Work out the finished part from the listing and answer in its coordinate system (mm). Round coordinates to 2 decimals unless told otherwise and drop trailing zeros.
from build123d import *

# Parameters (mm, degrees)
F1_DEPTH = 200
F4_T     = -0.6
F3_W     = 0.2
F3_H     = 14
F5_DEPTH = 25
F6_W     = 0.2
F6_H     = 14
F7_DEPTH = 25
F8_R     = 0.4


with BuildPart() as f1:
    # F0 (on Right) → F1 (new body)
    with BuildSketch(Plane.YZ):
        with BuildLine():
            add(Edge.make_bspline(
                [(18.4494327754, -3.8520128001), (15.5609515421, -0.4847487874), (8.1340167717, 2.2164674432), (-12.2966120419, 0.5504568669), (-24.9624218007, -2.9072897866), (-31.5505672246, -3.8520128001)],
                knots=[0, 0, 0, 0, 0.2747109337, 0.6355042516, 1, 1, 1, 1], degree=3))
            Line((-31.5505672246, -3.8520128001), (18.4494327754, -3.8520128001))
        make_face()
    extrude(amount=F1_DEPTH)


with BuildPart() as f1_1:
    # F2: moved
    add(f1.part.moved(Location((-100, 0, 16.3))))

    # F4
    f4_openings = [f1_1.faces().sort_by_distance(p)[0] for p in [
        (100, -2.298769, 14.541602),
        (-100, -2.298769, 14.541602),
    ]]
    offset(amount=F4_T, openings=f4_openings)

    # F3 (on face) → F5 (cut)
    with BuildSketch(Plane(origin=(0, 0, 12.4479871999), x_dir=(1, 0, 0), z_dir=(0, 0, -1))):
        with Locations((89.8042006254, 24.5505672246)):
            Rectangle(F3_W, F3_H)
        with Locations((-89.8042006254, 24.5505672246)):
            Rectangle(F3_W, F3_H)
    extrude(amount=-F5_DEPTH, mode=Mode.SUBTRACT)

    # F6 (on face) → F7 (cut)
    with BuildSketch(Plane(origin=(0, 0, 12.4479871999), x_dir=(1, 0, 0), z_dir=(0, 0, -1))):
        with Locations((-20.9039503872, 24.5505672246)):
            Rectangle(F6_W, F6_H)
        with Locations((20.9039503872, 24.5505672246)):
            Rectangle(F6_W, F6_H)
    extrude(amount=-F7_DEPTH, mode=Mode.SUBTRACT)

    # F8
    f8_edges = [f1_1.edges().sort_by_distance(p)[0] for p in [
        (0, 18.449433, 12.447987),
    ]]
    fillet(f8_edges, radius=F8_R)


solid = f1_1.part
Q1. The mould has two halves that part along Z. Classify faces 1 (the face through (-1, -7, 12.448)), 2 (the face through (-1, -4, 13.048)), 3 (the face through (-100, -5.1, 12.8)): +Z half, -Z half, draft (parallel to the pull), parting line (faces both ways), or undercut.
Q2. Find section A-A (y = -21). Count the separate pieces of the cut face and the enclosed holes in it, plus the area to 3 significant figures.
Q3. Given pin 1 (0.8 mm diameter, centred on y = -28, z = 14.5, fed in from +X); pin 2 (3 mm diameter, centred on y = -24.5, z = 14, fed in from -X); pin 3 (10 mm diameter, centred on x = -44.5, y = -23.5, fed in from +Z); pin 4 (1 mm diameter, centred on x = 47, z = 14.5, fed in from +Y), each flat-ended and moving along its own axis, determine where each tip first touches the part or whether it passes through.
Q4. Find the intervals of material crossed by L1, parallel to Z at x = 77, y = 4.5; L2, parallel to Z at x = -42, y = -6.5; L3, parallel to Z at x = 35, y = -25.5, in increasing order.
Report:
1. face 1: -Z half
1. face 2: undercut
1. face 3: draft
2. separate pieces: 10
2. enclosed holes: 0
2. area: 242 mm2
3. pin 1: passes through
3. pin 2: stops at x = -100
3. pin 3: stops at z = 14.98
3. pin 4: stops at y = 16.92
4. L1: z = 12.45 to 13.05, 17.08 to 17.68
4. L2: z = 12.45 to 13.05, 16.45 to 17.05
4. L3: z = 12.45 to 13.51
